```python
from build123d import *

# Parameters (mm, degrees)
F0_R         = 4.699
F1_DEPTH     = 1.6256
F3_DEPTH     = 3.81
F4_R         = 6.858
F5_DEPTH     = 2.54
F6_R         = 4.25
F7_DEPTH     = 50.8
F8_T8_DEPTH  = 7.2082729301
F8_S9_R      = 6.858
F8_T10_DEPTH = 5
F8_T14_DEPTH = 7.2082729301
F8_S15_R     = 6.858
F8_T16_DEPTH = 5
F8_T22_DEPTH = 7.2082729301
F8_S23_R     = 6.858
F8_T24_DEPTH = 5
F8_T28_DEPTH = 7.2082729301
F8_S29_R     = 6.858
F8_T30_DEPTH = 5


# Not quite as in the source:
# - a fillet or chamfer that OpenCascade refuses, or shapes differently, is made with other operations: its cross-section is extruded or revolved along the edge and cut away or added


with BuildPart() as f1:
    # F0 (on Top) → F1 (new body)
    with BuildSketch(Plane.XY):
        with BuildLine():
            Line((6.858, -5.2486504932), (6.858, 5.2486504932))
            ThreePointArc((6.858, 5.2486504932), (0, 8.636), (-6.858, 5.2486504932))
            Line((-6.858, 5.2486504932), (-6.858, -5.2486504932))
            ThreePointArc((-6.858, -5.2486504932), (0, -8.636), (6.858, -5.2486504932))
        make_face()
        Circle(F0_R, mode=Mode.SUBTRACT)
    extrude(amount=-F1_DEPTH)

    # F2 (on face) → F3 (join)
    with BuildSketch(Plane.XY):
        with BuildLine():
            ThreePointArc((-6.858, 0), (0, -6.858), (6.858, 0))
            ThreePointArc((6.858, 0), (0, 6.858), (-6.858, 0))
        make_face()
        with BuildLine():
            ThreePointArc((0, 3.683), (3.683, 0), (0, -3.683))
            ThreePointArc((0, -3.683), (-3.683, 0), (0, 3.683))
        make_face(mode=Mode.SUBTRACT)
    extrude(amount=F3_DEPTH)

    # F4 (on face) → F5 (join)
    with BuildSketch(Plane.XY.offset(3.81)):
        Circle(F4_R)
        with BuildLine():
            Line((-0.508, 3.1340965205), (-0.508, -3.1340965205))
            ThreePointArc((-0.508, -3.1340965205), (-3.175, 0), (-0.508, 3.1340965205))
        make_face(mode=Mode.SUBTRACT)
        with BuildLine():
            ThreePointArc((0.508, 3.1340965205), (3.175, 0), (0.508, -3.1340965205))
            Line((0.508, -3.1340965205), (0.508, 3.1340965205))
        make_face(mode=Mode.SUBTRACT)
    extrude(amount=F5_DEPTH)

    # F6 (on face) → F7 (join)
    with BuildSketch(Plane.XY.offset(6.35)):
        Circle(F6_R)
        with BuildLine():
            Line((-0.508, 3.1340965205), (-0.508, -3.1340965205))
            ThreePointArc((-0.508, -3.1340965205), (-3.175, 0), (-0.508, 3.1340965205))
        make_face(mode=Mode.SUBTRACT)
        with BuildLine():
            ThreePointArc((0.508, 3.1340965205), (3.175, 0), (0.508, -3.1340965205))
            Line((0.508, -3.1340965205), (0.508, 3.1340965205))
        make_face(mode=Mode.SUBTRACT)
    extrude(amount=F7_DEPTH)

    # F8: chamfer of 0.762 on 5 edges, made by hand

    # F8_s1 → F8_t2 (revolve)
    with BuildSketch(Plane.XZ):
        Polygon((4.25, 7.112), (5.012, 6.35), (4.25, 6.35), align=None)
    revolve(axis=Axis((0, 0, 6.35), (0, 0, 1)))

    # F8_s3 → F8_t4 (revolve, cut)
    with BuildSketch(Plane.XZ):
        Polygon((6.858, 5.588), (6.096, 6.35), (6.858, 6.35), align=None)
    revolve(axis=Axis((0, 0, 6.35), (0, 0, 1)), mode=Mode.SUBTRACT)


with BuildPart() as f8_tool6:
    # F8_s7 → F8_t8 (new body)
    with BuildSketch(Plane.XZ.offset(-7.2082729301)):
        Polygon((-6.096, 0), (-6.858, -0.762), (-6.858, 0), align=None)
    extrude(amount=F8_T8_DEPTH)

    # F8_s9 → F8_t10 (cut, symmetric)
    with BuildSketch(Plane.XY.offset(-0.4)):
        Circle(F8_S9_R)
    extrude(amount=F8_T10_DEPTH, both=True, mode=Mode.SUBTRACT)


with BuildPart() as f1_1:
    add(f1.part)

    # F8_t5: cut F8_tool6
    add(f8_tool6.part, mode=Mode.SUBTRACT)


with BuildPart() as f8_tool12:
    # F8_s13 → F8_t14 (new body)
    with BuildSketch(Plane.XZ):
        Polygon((6.858, -0.762), (6.096, 0), (6.858, 0), align=None)
    extrude(amount=-F8_T14_DEPTH)

    # F8_s15 → F8_t16 (cut, symmetric)
    with BuildSketch(Plane.XY.offset(-0.4)):
        Circle(F8_S15_R)
    extrude(amount=F8_T16_DEPTH, both=True, mode=Mode.SUBTRACT)


with BuildPart() as f1_2:
    add(f1_1.part)

    # F8_t11: cut F8_tool12
    add(f8_tool12.part, mode=Mode.SUBTRACT)

    # F8_s17 → F8_t18 (revolve, cut)
    with BuildSketch(Plane.XZ):
        Polygon((4.25, 56.388), (3.488, 57.15), (4.25, 57.15), align=None)
    revolve(axis=Axis((0, 0, 57.15), (0, 0, 1)), mode=Mode.SUBTRACT)


with BuildPart() as f8_tool20:
    # F8_s21 → F8_t22 (new body)
    with BuildSketch(Plane.XZ.offset(7.2082729301)):
        Polygon((6.858, -0.762), (6.096, 0), (6.858, 0), align=None)
    extrude(amount=-F8_T22_DEPTH)

    # F8_s23 → F8_t24 (cut, symmetric)
    with BuildSketch(Plane.XY.offset(-0.4)):
        Circle(F8_S23_R)
    extrude(amount=F8_T24_DEPTH, both=True, mode=Mode.SUBTRACT)


with BuildPart() as f1_3:
    add(f1_2.part)

    # F8_t19: cut F8_tool20
    add(f8_tool20.part, mode=Mode.SUBTRACT)


with BuildPart() as f8_tool26:
    # F8_s27 → F8_t28 (new body)
    with BuildSketch(Plane.XZ):
        Polygon((-6.096, 0), (-6.858, -0.762), (-6.858, 0), align=None)
    extrude(amount=F8_T28_DEPTH)

    # F8_s29 → F8_t30 (cut, symmetric)
    with BuildSketch(Plane.XY.offset(-0.4)):
        Circle(F8_S29_R)
    extrude(amount=F8_T30_DEPTH, both=True, mode=Mode.SUBTRACT)


with BuildPart() as f1_4:
    add(f1_3.part)

    # F8_t25: cut F8_tool26
    add(f8_tool26.part, mode=Mode.SUBTRACT)


solid = f1_4.part
```
Design review of the part built by this model. Coordinates are the model's own, in mm. A direction names the side the tool comes from. Round coordinates to 2 decimals unless told otherwise and drop trailing zeros. Order: outer loops, then holes, each group sorted by start corner. A loop starts at its lowest first (then second) coordinate and runs counter-clockwise, first axis right, second up. Notation, with made-up numbers: (75, 5) - (107, 5) arc R21 cw to (107, 20) - close; hole circle Ø10 at (-3, -26). An arc over 180 degrees is marked (long way). Return JSON: item names as keys, results as strings.
Q1. Consider section C-C on y = -1.5. Give the number of separate pieces and of enclosed holes in the cut face, plus the area to 3 significant figures.
Computed values:
{"separate pieces": "3", "enclosed holes": "0", "area": "226 mm2"}
Q2. Consider section A-A on z = 47. Write out the cut boundary in (x, y) (3 decimals).
Computed values:
{"outline": "circle Ø8.5 at (0, 0); hole (-0.508, -3.134) - (-0.508, 3.134) arc R3.175 ccw to start; hole (0.508, -3.134) arc R3.175 ccw to (0.508, 3.134) - close"}
Q3. Machinability: for faces 1 (the flat face through (-0.5, -7.1, 0)), 2 (the cylindrical face through (3.267, -1.699, 1.878)), 3 (the flat face through (0.508, 0, 30)), 4 (the flat face through (-0.1, 7.1, 0)), which of the approach directions +Z, -Z, +X, -X, +Y, -Y give a long, thin tool a straight path to every point of the face, cutting with its end or side? Answer none if there is none.
Computed values:
{"face 1": "+Z, -Y", "face 2": "-Z", "face 3": "+Z, -Z", "face 4": "+Z, +Y"}
Q4. For pin 1 Ø6 at (y, z) = (-5, 22.5) entering from -X; pin 2 Ø7 at (y, z) = (1, 32) entering from +X; pin 3 Ø5 at (y, z) = (1, 39) entering from -X; pin 4 Ø1.5 at (x, z) = (-5.5, 38.5) entering from +Y, all flat-tipped, find the tip position at first contact; note any pin that passes through.
Computed values:
{"pin 1": "stops at x = -3.75", "pin 2": "stops at x = 4.25", "pin 3": "stops at x = -4.25", "pin 4": "passes through"}
Q5. Wall thickness on L1, parallel to X at y = 2.75, z = 19; L2, parallel to Y at x = 0, z = -0.8; L3, parallel to X at y = 0, z = 1.75: over which ranges is each line inside the solid? List them lowest first. Write a range as [from, to].
Computed values:
{"L1": "x = [-3.24, -1.59], [-0.51, 0.51], [1.59, 3.24]", "L2": "y = [-8.64, -4.7], [4.7, 8.64]", "L3": "x = [-6.86, -3.68], [3.68, 6.86]"}
Q6. Consider section B-B on x = 0. Write out the cut boundary in (y, z), plus the area to 3 significant figures.
Computed values:
{"outline": "(-8.64, -1.63) - (-4.7, -1.63) - (-4.7, 0) - (-3.68, 0) - (-3.68, 3.81) - (3.68, 3.81) - (3.68, 0) - (4.7, 0) - (4.7, -1.63) - (8.64, -1.63) - (8.64, 0) - (6.86, 0) - (6.86, 5.59) - (6.1, 6.35) - (5.01, 6.35) - (4.25, 7.11) - (4.25, 56.39) - (3.49, 57.15) - (-3.49, 57.15) - (-4.25, 56.39) - (-4.25, 7.11) - (-5.01, 6.35) - (-6.1, 6.35) - (-6.86, 5.59) - (-6.86, 0) - (-8.64, 0) - close", "area": "503 mm2"}
